Part model, mm, in its own coordinate system. A direction names the side the tool comes from. Round coordinates to 2 decimals unless told otherwise and drop trailing zeros. Loops run counter-clockwise (first coordinate to the right, second up) from the corner with the lowest first, then second, coordinate; pieces in that order, holes last. Notation, with made-up numbers: (54, -4) -> (72, -4) arc R24 ccw to (72, 23) -> close; hole circle Ø8 at (87, 63). An arc over 180 degrees is marked (long way). Answer as CSV lines item,"result".
from build123d import *

# Parameters (mm, degrees)
EXTRUDE_1_DEPTH     = 9.6
SKETCH_2_W          = 14.6
SKETCH_2_H          = 8.5
CUT_EXTRUDE_1_DEPTH = 4.8
SKETCH_3_W          = 6
SKETCH_3_H          = 8.5
CUT_EXTRUDE_2_DEPTH = 2.5


with BuildPart() as part:
    # 草图1 → 凸台-拉伸1 (new body)
    with BuildSketch(Plane.XY):
        Polygon((-7.3, 0), (-7.3, 38.5), (7.3, 38.5), (7.3, 0), (7.3, -8.5), (-7.3, -8.5), align=None)
    extrude(amount=EXTRUDE_1_DEPTH)

    # 草图2 → 切除-拉伸1 (cut)
    with BuildSketch(Plane.XY.offset(9.6)):
        with Locations((0, -4.25)):
            Rectangle(SKETCH_2_W, SKETCH_2_H)
    extrude(amount=-CUT_EXTRUDE_1_DEPTH, mode=Mode.SUBTRACT)

    # 草图3 → 切除-拉伸2 (cut)
    with BuildSketch(Plane.XY.offset(4.8)):
        with Locations((0, -4.25)):
            Rectangle(SKETCH_3_W, SKETCH_3_H)
    extrude(amount=-CUT_EXTRUDE_2_DEPTH, mode=Mode.SUBTRACT)


solid = part.part
Q1. Saw through at C-C, the plane y = -4.5. Write the cut outline in (x, z).
Geometry results:
outline,"(-7.3, 0) -> (7.3, 0) -> (7.3, 4.8) -> (3, 4.8) -> (3, 2.3) -> (-3, 2.3) -> (-3, 4.8) -> (-7.3, 4.8) -> close"
Q2. Saw through at B-B, the plane x = 5. Write the cut outline in (y, z).
Geometry results:
outline,"(-8.5, 0) -> (38.5, 0) -> (38.5, 9.6) -> (0, 9.6) -> (0, 4.8) -> (-8.5, 4.8) -> close"
Q3. Saw through at A-A, the plane z = 3.25. Write the cut outline in (x, y), then the cut area to 3 significant figures.
Geometry results:
outline,"(-7.3, -8.5) -> (-3, -8.5) -> (-3, 0) -> (3, 0) -> (3, -8.5) -> (7.3, -8.5) -> (7.3, 38.5) -> (-7.3, 38.5) -> close"
area,"635 mm2"
Q4. Which spindle directions (+Z, -Z, +X, -X, +Y, -Y) get a long thin tool onto all of the face, cutting with end or side? Do faces 1 (the face through (0, 15, 0)), 2 (the face through (0, -4, 2.3)), 3 (the face through (-5, -4, 4.8)). Say none if no direction does.
Geometry results:
face 1,"-Z, +X, -X, +Y, -Y"
face 2,"+Z, -Y"
face 3,"+Z, +X, -X, -Y"
Q5. Two-plate mould, pull along X, no slides. Class faces 4 (the face through (0, 20, 9.6)), 5 (the face through (0, 0, 7)), 6 (the face through (-7.3, 15, 5)): pulls with the +X half, pulls with the -X half, needs draft (parallel to the pull), parting line crosses it, or undercut.
Geometry results:
face 4,"needs draft"
face 5,"undercut"
face 6,"pulls with the -X half"
Q6. Drill centre lines: line 1 along X through (y, z) = (-1, 4); line 2 along Y through (x, z) = (5, 8.75). Where is each one in solid material? Low to high.
Geometry results:
line 1,"-7.3 to -3, 3 to 7.3"
line 2,"0 to 38.5"
Q7. Saw through at D-D, the plane x = -2. Write the cut outline in (y, z).
Geometry results:
outline,"(-8.5, 0) -> (38.5, 0) -> (38.5, 9.6) -> (0, 9.6) -> (0, 2.3) -> (-8.5, 2.3) -> close"
Q8. Drop flat-ended pins along their axis: P1, Ø1, axis at x = -0.5, y = -2, coming from the +Z side; P2, Ø1.3, axis at x = -6, y = -4, coming from the +Z side. Give the stop position or say it passes through.
Geometry results:
P1,"z = 2.3"
P2,"z = 4.8"
